The model under review builds one solid part; all positions refer to its coordinate system, in mm. A direction names the side the tool comes from. Coordinates: 2 decimals unless noted, no trailing zeros. Order: outer loops, then holes, each group sorted by start corner. A loop starts at its lowest first (then second) coordinate and runs counter-clockwise, first axis right, second up. Notation, with made-up numbers: M -6.75,48.5 L 26.25,48.5 A26 ccw 26.25,73.5 Z; hole C -35.75,40 d6. An arc over 180 degrees is marked long. One line per item, written item: value.
```python
from build123d import *

# Parameters (mm, degrees)
BOSS_EXTRUDE1_DEPTH = 20


with BuildPart() as part:
    # Sketch1 → Boss-Extrude1 (new body)
    with BuildSketch(Plane(origin=(0, 0, 0), x_dir=(1, 0, 0), z_dir=(0, 1, 0))):
        Polygon((0, 404.145188433), (-350, -202.072594216), (350, -202.072594216), align=None)
        Polygon((0, 381.051177665), (-330, -190.525588833), (330, -190.525588833), align=None, mode=Mode.SUBTRACT)
    extrude(amount=BOSS_EXTRUDE1_DEPTH)


solid = part.part
```
(1) We need section A-A, the plane y = 14.5. State the section outline as (x, z) points, plus the area to 3 significant figures.
Geometry results:
outline: M -350,202.07 L 0,-404.15 L 350,202.07 Z; hole M -330,190.53 L 0,-381.05 L 330,190.53 Z
area: 23,600 mm2
(2) Mouldability with a two-part tool opening along X and no side actions: class faces 3 (the flat face through (-131, 0, -170)), 4 (the flat face through (-5, 10, 190.526)), 5 (the flat face through (-172.55, 9.86, -105.28)) as +X half, -X half, draft (parallel to the pull), parting line (faces both ways), or undercut.
Geometry results:
face 3: draft
face 4: undercut
face 5: -X half
(3) We need section C-C, the plane z = -90.5. State the section outline as (x, y) points.
Geometry results:
outline: M -181.08,0 L -167.75,0 L -167.75,20 L -181.08,20 Z; M 167.75,0 L 181.08,0 L 181.08,20 L 167.75,20 Z
(4) We need section B-B, the plane x = 81. State the section outline as (y, z) points, plus the area to 3 significant figures.
Geometry results:
outline: M 0,-263.85 L 20,-263.85 L 20,-240.76 L 0,-240.76 Z; M 0,190.53 L 20,190.53 L 20,202.07 L 0,202.07 Z
area: 693 mm2
(5) For L1, parallel to Z at x = 60, y = 11.75; L2, parallel to X at y = 11.5, z = -360.5; L3, parallel to X at y = 5.5, z = 99.5, list the stretches that pass through material, from the lowest coordinate up.
Geometry results:
L1: z = -300.22 to -277.13, 190.53 to 202.07
L2: x = -25.2 to -11.87, 11.87 to 25.2
L3: x = -290.78 to -277.45, 277.45 to 290.78
(6) Insertion check: pin 1 Ø5 at (y, z) = (6.5, 17.5) entering from +X; pin 2 Ø10 at (x, y) = (25, 6) entering from -Z; pin 3 Ø10 at (y, z) = (13, -94.5) entering from -X. Each pin has a flat end and moves straight along its axis. Give the tip position at first contact, or say it passes through.
Geometry results:
pin 1: stops at x = 244.88
pin 2: stops at z = -369.5
pin 3: stops at x = -181.66
(7) Tool access review of faces 1 (the flat face through (-162.69, 9.86, -99.26)), 2 (the flat face through (-131, 20, -170)): name each direction out of +Z, -Z, +X, -X, +Y, -Y from which nothing blocks a thin tool from reaching the whole face with its end or side.
Geometry results:
face 1: +Y, -Y
face 2: +Z, -Z, +X, -X, +Y
